from build123d import *

# Parameters (mm, degrees)
BOSS_EXTRUDE1_DEPTH      = 3
SKETCH5_W                = 3.213765407
SKETCH5_H                = 0.4
BOSS_EXTRUDE2_DEPTH      = 3.9
CHAMFER2_SIZE            = 0.25
SKETCH6_R                = 0.8
CUT_EXTRUDE1_DEPTH       = 21.612860064
FILLET1_R                = 0.5
SKETCH7_R                = 1.2
CUT_EXTRUDE2_DEPTH       = 15.730919863
BOSS_EXTRUDE5_DEPTH      = 3.2
BOSS_EXTRUDE5_DEPTH_BACK = 3.4
SKETCH11_R               = 1.2
SKETCH12_R               = 0.3
CUT_EXTRUDE3_DEPTH       = 15.898322053
CUT_EXTRUDE4_DEPTH       = 2
CUT_EXTRUDE4_DEPTH_BACK  = 2


with BuildPart() as part:
    # Sketch1 → Boss-Extrude1 (new, symmetric)
    with BuildSketch(Plane(origin=(0, 0, 0), x_dir=(0, 0, -1), z_dir=(1, 0, 0))):
        Polygon((10, 4.4), (0, 4.4), (-1.147622848, 5.1), (-10, 5.1), (-10, -5.1), (-6.5, -5.1), (-6.1, -5.5), (-3.4, -5.5), (-3, -5.1), (3, -5.1), (3.4, -5.5), (6.1, -5.5), (6.5, -5.1), (10, -5.1), align=None)
    extrude(amount=BOSS_EXTRUDE1_DEPTH, both=True)

    # Sketch5 → Boss-Extrude2 (add)
    with BuildSketch(Plane.XZ.offset(5.1)):
        with Locations((0.02921605, 8.1)):
            Rectangle(SKETCH5_W, SKETCH5_H)
        with Locations((0.02921605, -0.7)):
            Rectangle(SKETCH5_W, SKETCH5_H)
        with Locations((0.02921605, -8)):
            Rectangle(SKETCH5_W, SKETCH5_H)
    extrude(amount=BOSS_EXTRUDE2_DEPTH)

    # Chamfer2
    chamfer2_edges = [part.edges().sort_by_distance(p)[0] for p in [
        (-1.577666654, -9, 8.1),
        (1.636098753, -9, 8.1),
        (-1.577666654, -9, -0.7),
        (1.636098753, -9, -0.7),
        (-1.577666654, -9, -8),
        (1.636098753, -9, -8),
    ]]
    chamfer(chamfer2_edges, length=CHAMFER2_SIZE)

    # Sketch6 → Cut-Extrude1 (cut, through all)
    with BuildSketch(Plane.XY.offset(8.3)):
        with Locations((0, -7.76874139)):
            Circle(SKETCH6_R)
    extrude(amount=-CUT_EXTRUDE1_DEPTH, mode=Mode.SUBTRACT)

    # Fillet1
    fillet1_edges = [part.edges().sort_by_distance(p)[0] for p in [
        (0, -5.1, 10),
        (0, 5.1, 10),
        (0, 4.4, -10),
        (0, -5.1, -10),
    ]]
    fillet(fillet1_edges, radius=FILLET1_R)

    # Sketch7 → Cut-Extrude2 (cut, through all)
    with BuildSketch(Plane(origin=(3, 0, 0), x_dir=(0, 0, -1), z_dir=(1, 0, 0))):
        with Locations((-4.75, -2.6)):
            Circle(SKETCH7_R)
        with Locations((4.75, -2.6)):
            Circle(SKETCH7_R)
    extrude(amount=-CUT_EXTRUDE2_DEPTH, mode=Mode.SUBTRACT)

    # Sketch11 → Boss-Extrude5 (add, two sides: drawn at the far end of the back side and taken through both)
    # profile 1 of 2: a face of its own
    with BuildSketch(Plane(origin=(0, 0, 0), x_dir=(0, 0, -1), z_dir=(1, 0, 0)).offset(-BOSS_EXTRUDE5_DEPTH_BACK)):
        with BuildLine():
            Line((-6.85, -4.453368072), (-2.65, -4.453368072))
            Line((-2.65, -4.453368072), (-2.65, -2.6))
            ThreePointArc((-2.65, -2.6), (-4.75, -0.5), (-6.85, -2.6))
            Line((-6.85, -2.6), (-6.85, -4.453368072))
        make_face()
        with Locations((-4.75, -2.6)):
            Circle(SKETCH11_R, mode=Mode.SUBTRACT)
    # profile 2 of 2: a face of its own
    with BuildSketch(Plane(origin=(0, 0, 0), x_dir=(0, 0, -1), z_dir=(1, 0, 0)).offset(-BOSS_EXTRUDE5_DEPTH_BACK)):
        with BuildLine():
            Line((2.678191921, -4.453368072), (6.878191921, -4.453368072))
            Line((6.878191921, -4.453368072), (6.878191921, -2.6))
            ThreePointArc((6.878191921, -2.6), (4.994944522, -0.485951033), (2.678191921, -2.113366526))
            Line((2.678191921, -2.113366526), (2.678191921, -4.453368072))
        make_face()
        with Locations((4.75, -2.6)):
            Circle(SKETCH11_R, mode=Mode.SUBTRACT)
    extrude(amount=BOSS_EXTRUDE5_DEPTH + BOSS_EXTRUDE5_DEPTH_BACK)

    # Sketch12 → Cut-Extrude3 (cut, through all)
    with BuildSketch(Plane(origin=(3, 0, 0), x_dir=(0, 0, -1), z_dir=(1, 0, 0))):
        with Locations((-6.3, 4.201970351)):
            Circle(SKETCH12_R)
    extrude(amount=-CUT_EXTRUDE3_DEPTH, mode=Mode.SUBTRACT)

    # Sketch13 → Cut-Extrude4 (cut, two sides: drawn at the far end of the back side and taken through both)
    with BuildSketch(Plane(origin=(0, 0, 0), x_dir=(0, 0, -1), z_dir=(1, 0, 0)).offset(-CUT_EXTRUDE4_DEPTH_BACK)):
        Polygon((-6.6, 4.201970351), (-6.6, 5.1), (-5.759373681, 5.1), (-6, 4.201970351), align=None)
    extrude(amount=CUT_EXTRUDE4_DEPTH + CUT_EXTRUDE4_DEPTH_BACK, mode=Mode.SUBTRACT)


solid = part.part
Could you check a few things on this model? Use its own coordinates, in mm. A direction names the side the tool comes from. Coordinates: 2 decimals unless noted, no trailing zeros. Write each loop counter-clockwise with the first axis right and the second up, starting at its lowest first coordinate (ties: lowest second). Pieces come first, ordered by that corner, then holes. Notation, with made-up numbers: (-10.75, 32.25) - (26.25, 32.25) arc R21 cw to (26.25, 69.25) - close; hole circle Ø6 at (39, 46). An arc over 180 degrees is marked (long way). Put each result on its own line as item: value. Start each with the question number.
Q1. I want a section at D-D on x = 0. Count the separate pieces of the cut face and the enclosed holes in it, plus the area to 3 significant figures.
Q2. Thinking about a two-plate mould opening in Z: for faces 1 (the flat face through (0, -5.1, 7.7)), 2 (the flat face through (0, -5.5, 5)), 3 (the flat face through (-3.4, -4, -4)), 4 (the flat face through (0, -6.6, 8.3)), which applies, pulls with the +Z half, pulls with the -Z half, needs draft (parallel to the pull), parting line crosses it, or undercut?
Q3. Which directions (+Z, -Z, +X, -X, +Y, -Y) give clear straight access to the entire face, cutting with the end or side of a thin tool? Please do faces 5 (the flat face through (0, -6.6, -0.5)), 6 (the cylindrical face through (-3.2, -0.49, -5.04)), 7 (the flat face through (0, 4.4, -5)).
Q4. Please list where these lines run through material, in increasing order: L1, parallel to Z at x = -1.25, y = -7.5; L2, parallel to Y at x = 0, z = -7.95; L3, parallel to Z at x = -1.5, y = -2.75.
Q5. I'm going to push flat-ended pins straight in: P1, Ø1.5, axis at y = -2.5, z = -5, coming from the -X side; P2, Ø3.5, axis at x = 0, y = -7, coming from the +Z side; P3, Ø0.8, axis at x = 1, z = 4, coming from the -Y side. Where does each tip first touch, or does it pass through?
Q6. I want a section at A-A on z = 4.75. Write out the boundary of the cut face in (x, y), plus the area to 3 significant figures.
Q7. I want a section at B-B on x = -2.5. Write out the boundary of the cut face in (y, z), plus the area to 3 significant figures.
Q8. I want a section at C-C on y = -7.5. Write out the boundary of the cut face in (x, z), plus the area to 3 significant figures.
Checks:
1. separate pieces: 4
1. enclosed holes: 2
1. area: 192 mm²
2. face 1: undercut
2. face 2: undercut
2. face 3: needs draft
2. face 4: pulls with the +Z half
3. face 5: +X, -X, -Y
3. face 6: -X, +Y
3. face 7: -Z, +X, -X, +Y
4. L1: -8.2 to -7.8, -0.9 to -0.5, 7.9 to 8.3
4. L2: -9 to -8.57, -6.97 to 4.4
4. L3: -10 to -5.94, -3.56 to 3.56, 5.94 to 10
5. P1: through
5. P2: z = 8.3
5. P3: y = -5.5
6. outline: (-3.4, -4.45) - (-3, -4.45) - (-3, -5.5) - (3, -5.5) - (3, -4.45) - (3.2, -4.45) - (3.2, -3.8) - (-3.4, -3.8) - close; (-3.4, -1.4) - (3.2, -1.4) - (3.2, -0.5) - (3, -0.5) - (3, 5.1) - (-3, 5.1) - (-3, -0.5) - (-3.4, -0.5) - close
6. area: 50.1 mm²
7. outline: (-5.5, -6.1) - (-5.1, -6.5) - (-5.1, -9.5) arc R0.5 ccw to (-4.6, -10) - (3.9, -10) arc R0.5 ccw to (4.4, -9.5) - (4.4, 0) - (5.1, 1.15) - (5.1, 9.5) arc R0.5 ccw to (4.6, 10) - (-4.6, 10) arc R0.5 ccw to (-5.1, 9.5) - (-5.1, 6.5) - (-5.5, 6.1) - (-5.5, 3.4) - (-5.1, 3) - (-5.1, -3) - (-5.5, -3.4) - close; hole circle Ø2.4 at (-2.6, -4.75); hole circle Ø2.4 at (-2.6, 4.75); hole circle Ø0.6 at (4.2, 6.3)
7. area: 190 mm²
8. outline: (-1.58, -8.2) - (-0.75, -8.2) - (-0.75, -7.8) - (-1.58, -7.8) - close; (-1.58, -0.9) - (-0.75, -0.9) - (-0.75, -0.5) - (-1.58, -0.5) - close; (-1.58, 7.9) - (-0.75, 7.9) - (-0.75, 8.3) - (-1.58, 8.3) - close; (0.75, -8.2) - (1.64, -8.2) - (1.64, -7.8) - (0.75, -7.8) - close; (0.75, -0.9) - (1.64, -0.9) - (1.64, -0.5) - (0.75, -0.5) - close; (0.75, 7.9) - (1.64, 7.9) - (1.64, 8.3) - (0.75, 8.3) - close
8. area: 2.05 mm²
